Input: part model. Units: mm. Frame: model coordinates. A direction names the side the tool comes from. Give positions to 0.01 mm unless a question says otherwise; leave off trailing zeros. Write each loop counter-clockwise with the first axis right and the second up, starting at its lowest first coordinate (ties: lowest second). Pieces come first, ordered by that corner, then holes. Notation, with made-up numbers: (-3, 25.25) - (14, 25.25) arc R13 cw to (14, 43.25) - close; hole circle Ø4 at (34, 15.5). An arc over 180 degrees is marked (long way). Answer as CSV lines item,"result".
```python
from build123d import *

# Parameters (mm, degrees)
EXTRUDE_1_DEPTH = 1.4


with BuildPart() as part:
    # Эскиз1 → Бобышка-Вытянуть1 (new, symmetric)
    with BuildSketch(Plane.XY):
        Polygon((-31.142857143, -2.8), (13.257142857, -2.8), (13.257142857, 1.12), (18.857142857, 1.12), (18.857142857, 5.04), (-31.142857143, 5.04), (-31.142857143, 2.24), (-33.942857143, 2.24), (-33.942857143, 0), (-33.942857143, -2.8), align=None)
    extrude(amount=EXTRUDE_1_DEPTH, both=True)


solid = part.part
```
Item 1: Cut plane C-C on y = 4.25. Return the cut outline in (x, z).
The answers:
outline,"(-31.14, -1.4) - (18.86, -1.4) - (18.86, 1.4) - (-31.14, 1.4) - close"
Item 2: Cut plane B-B on y = -0.75. Return the cut outline in (x, z), plus the area to 3 significant figures.
The answers:
outline,"(-33.94, -1.4) - (13.26, -1.4) - (13.26, 1.4) - (-33.94, 1.4) - close"
area,"132 mm²"
Item 3: Cut plane A-A on z = -0.6. Return the cut outline in (x, y).
The answers:
outline,"(-33.94, -2.8) - (13.26, -2.8) - (13.26, 1.12) - (18.86, 1.12) - (18.86, 5.04) - (-31.14, 5.04) - (-31.14, 2.24) - (-33.94, 2.24) - close"
Item 4: Contact query for flat-ended pins moving along their axis: pin 1 (0.8 mm diameter, centred on y = 0, z = -0.5, fed in from +X); pin 2 (0.8 mm diameter, centred on y = 3, z = -0.5, fed in from -X); pin 3 (1.4 mm diameter, centred on x = 15.5, z = 0, fed in from -Y). Output: stop coordinate, or through.
The answers:
pin 1,"x = 13.26"
pin 2,"x = -31.14"
pin 3,"y = 1.12"
Item 5: Reachability of faces 1 (the face through (16, 1.12, 0)), 2 (the face through (-33.943, 0, 0)), 3 (the face through (-31.143, 4, 0)) from +Z, -Z, +X, -X, +Y, -Y: full face, straight path, thin tool, end or side. Return the list, or none.
The answers:
face 1,"+Z, -Z, +X, -Y"
face 2,"+Z, -Z, -X, +Y, -Y"
face 3,"+Z, -Z, -X, +Y"
Item 6: Ray query, line 1 (X direction, y = -1.25, z = 0.6); line 2 (X direction, y = 3.5, z = 0.8); line 3 (Y direction, x = 16, z = 0.6). Return the intervals inside material, ascending. Write a range as from..to.
The answers:
line 1,"-33.94..13.26"
line 2,"-31.14..18.86"
line 3,"1.12..5.04"
